```python
from build123d import *

# Parameters (mm, degrees)
CROQUIS1_W                     = 0.64
CROQUIS1_H                     = 0.64
SALIENTE_EXTRUIR1_DEPTH        = 2.54
SALIENTE_EXTRUIR2_DEPTH        = 8.54
SALIENTE_EXTRUIR2_DEPTH_BACK   = 3
CROQUIS3_W                     = 0.64
CROQUIS3_H                     = 0.64
SALIENTE_EXTRUIR2_2_DEPTH      = 8.54
SALIENTE_EXTRUIR2_2_DEPTH_BACK = 3
CHAFL_N1_SIZE                  = 0.2
CHAFL_N2_SIZE                  = 0.2
CROQUIS1_4_W                   = 11
CROQUIS1_4_H                   = 3
BOSS_EXTRUDE6_DEPTH            = 2.54
SKETCH6_W                      = 11
SKETCH6_H                      = 3
SKETCH6_R                      = 1
BOSS_EXTRUDE11_DEPTH           = 0.8
SKETCH7_W                      = 13
SKETCH7_H                      = 5
SKETCH7_W_2                    = 11
SKETCH7_H_2                    = 3
BOSS_EXTRUDE12_DEPTH           = 15
SKETCH8_W                      = 13
SKETCH8_H                      = 5
SKETCH8_R                      = 2
BOSS_EXTRUDE13_DEPTH           = 1
BOSS_EXTRUDE15_DEPTH           = 2
BOSS_EXTRUDE15_DEPTH_BACK      = 1.5
SKETCH9_R                      = 3
SKETCH9_R_2                    = 2
SKETCH10_W                     = 0.5
SKETCH10_H                     = 1.275200555
CUT_EXTRUDE2_DEPTH             = 3
BOSS_EXTRUDE20_DEPTH           = 3
CUT_EXTRUDE3_DEPTH             = 3
CUT_EXTRUDE5_DEPTH             = 18.878324866
CUT_EXTRUDE5_DEPTH_BACK        = 18.878324866


with BuildPart() as part:
    # Croquis1 → Saliente-Extruir1 (new body)
    # profile 1 of 2: a face of its own
    with BuildSketch(Plane(origin=(0, 0, 0), x_dir=(0, 0, -1), z_dir=(1, 0, 0))):
        Polygon((1.27, 0.595482683), (1.27, -0.595482683), (0.595482683, -1.27), (-0.595482683, -1.27), (-1.27, -0.595482683), (-1.27, 0.595482683), (-0.595482683, 1.27), (0.595482683, 1.27), align=None)
        Rectangle(CROQUIS1_W, CROQUIS1_H, mode=Mode.SUBTRACT)
    # profile 2 of 2: a face of its own
    with BuildSketch(Plane(origin=(0, 0, 0), x_dir=(0, 0, -1), z_dir=(1, 0, 0))):
        Polygon((3.135482683, 1.27), (3.81, 0.595482683), (3.81, -0.595482683), (3.135482683, -1.27), (1.944517317, -1.27), (1.27, -0.595482683), (1.27, 0.595482683), (1.944517317, 1.27), align=None)
        with Locations((2.54, 0)):
            Rectangle(CROQUIS1_W, CROQUIS1_H, mode=Mode.SUBTRACT)
    extrude(amount=SALIENTE_EXTRUIR1_DEPTH)

    # Mirror5: part across plane


with BuildPart() as body_2:
    # Croquis3 → Saliente-Extruir2 (new, two sides: drawn at the far end of the back side and taken through both)
    with BuildSketch(Plane(origin=(0, 0, 0), x_dir=(0, 0, -1), z_dir=(1, 0, 0)).offset(-SALIENTE_EXTRUIR2_DEPTH_BACK)):
        Rectangle(CROQUIS3_W, CROQUIS3_H)
    extrude(amount=SALIENTE_EXTRUIR2_DEPTH + SALIENTE_EXTRUIR2_DEPTH_BACK)

    # Chaflán1
    chafl_n1_edges = [body_2.edges().sort_by_distance(p)[0] for p in [
        (-3, 0, -0.32),
        (8.54, 0, 0.32),
        (8.54, -0.32, 0),
        (-3, 0.32, 0),
        (8.54, 0, -0.32),
        (8.54, 0.32, 0),
        (-3, 0, 0.32),
        (-3, -0.32, 0),
    ]]
    chamfer(chafl_n1_edges, length=CHAFL_N1_SIZE)


with BuildPart() as body_3:
    # Croquis3 → Saliente-Extruir2 2 (new, two sides: drawn at the far end of the back side and taken through both)
    with BuildSketch(Plane(origin=(0, 0, 0), x_dir=(0, 0, -1), z_dir=(1, 0, 0)).offset(-SALIENTE_EXTRUIR2_2_DEPTH_BACK)):
        with Locations((2.54, 0)):
            Rectangle(CROQUIS3_W, CROQUIS3_H)
    extrude(amount=SALIENTE_EXTRUIR2_2_DEPTH + SALIENTE_EXTRUIR2_2_DEPTH_BACK)

    # Chaflán2
    chafl_n2_edges = [body_3.edges().sort_by_distance(p)[0] for p in [
        (-3, 0, -2.86),
        (8.54, 0, -2.22),
        (8.54, -0.32, -2.54),
        (-3, 0.32, -2.54),
        (8.54, 0, -2.86),
        (8.54, 0.32, -2.54),
        (-3, 0, -2.22),
        (-3, -0.32, -2.54),
    ]]
    chamfer(chafl_n2_edges, length=CHAFL_N2_SIZE)


with BuildPart() as body_4:
    # Mirror3: mirrored copy
    add(body_2.part.mirror(Plane(origin=(2.54, 0, 1.27), x_dir=(1, 0, 0), z_dir=(0, 0, -1))))


with BuildPart() as body_5:
    # Mirror3 2: mirrored copy
    add(body_3.part.mirror(Plane(origin=(2.54, 0, 1.27), x_dir=(1, 0, 0), z_dir=(0, 0, -1))))


with BuildPart() as part_1:
    add(part.part)
    add(part.part.mirror(Plane(origin=(2.54, 0, 1.27), x_dir=(1, 0, 0), z_dir=(0, 0, -1))))


with BuildPart() as body_6:
    # Croquis1<4> → Boss-Extrude6 (new body)
    with BuildSketch(Plane(origin=(0, 0, 0), x_dir=(0, 0, -1), z_dir=(1, 0, 0))):
        with Locations((-1.27, 0)):
            Rectangle(CROQUIS1_4_W, CROQUIS1_4_H)
        Polygon((1.944517317, 1.27), (3.135482683, 1.27), (3.81, 0.595482683), (3.81, -0.595482683), (3.135482683, -1.27), (1.944517317, -1.27), (1.27, -0.595482683), (0.595482683, -1.27), (-0.595482683, -1.27), (-1.27, -0.595482683), (-1.27, 0.595482683), (-0.595482683, 1.27), (0.595482683, 1.27), (1.27, 0.595482683), align=None, mode=Mode.SUBTRACT)
    extrude(amount=BOSS_EXTRUDE6_DEPTH)

    # Combine5: cut body 2, body 3, body 4, body 5, part
    add(body_2.part, mode=Mode.SUBTRACT)
    add(body_3.part, mode=Mode.SUBTRACT)
    add(body_4.part, mode=Mode.SUBTRACT)
    add(body_5.part, mode=Mode.SUBTRACT)
    add(part_1.part, mode=Mode.SUBTRACT)

    # Sketch6 → Boss-Extrude11 (add)
    with BuildSketch(Plane.ZY):
        with Locations((1.27, 0)):
            Rectangle(SKETCH6_W, SKETCH6_H)
        with Locations((-2.54, 0)):
            Circle(SKETCH6_R, mode=Mode.SUBTRACT)
        with Locations((0, 0.013602928)):
            Circle(SKETCH6_R, mode=Mode.SUBTRACT)
        with Locations(Location((2.54, 0, 0), (0, 0, 180))):
            Circle(SKETCH6_R, mode=Mode.SUBTRACT)
        with Locations(Location((5.08, 0, 0), (0, 0, 180))):
            Circle(SKETCH6_R, mode=Mode.SUBTRACT)
    extrude(amount=BOSS_EXTRUDE11_DEPTH)

    # Sketch7 → Boss-Extrude12 (add)
    with BuildSketch(Plane(origin=(2.54, 0, 0), x_dir=(0, 0, -1), z_dir=(1, 0, 0))):
        with Locations((-1.27, 0)):
            Rectangle(SKETCH7_W, SKETCH7_H)
        with Locations((-1.27, 0)):
            Rectangle(SKETCH7_W_2, SKETCH7_H_2, mode=Mode.SUBTRACT)
    extrude(amount=-BOSS_EXTRUDE12_DEPTH)

    # Sketch8 → Boss-Extrude13 (add)
    with BuildSketch(Plane.ZY.offset(12.46)):
        with Locations((1.27, 0)):
            Rectangle(SKETCH8_W, SKETCH8_H)
        with Locations(Location((1.27, 0, 0), (0, 0, 131.409622109))):
            Circle(SKETCH8_R, mode=Mode.SUBTRACT)
    extrude(amount=BOSS_EXTRUDE13_DEPTH)

    # Sketch9 → Boss-Extrude15 (add, two sides: drawn at the far end of the back side and taken through both)
    with BuildSketch(Plane.ZY.offset(13.46).offset(-BOSS_EXTRUDE15_DEPTH_BACK)):
        with Locations(Location((1.27, 0, 0), (0, 0, 123.557309762))):
            Circle(SKETCH9_R)
        with Locations(Location((1.27, 0, 0), (0, 0, 131.409622109))):
            Circle(SKETCH9_R_2, mode=Mode.SUBTRACT)
    extrude(amount=BOSS_EXTRUDE15_DEPTH + BOSS_EXTRUDE15_DEPTH_BACK)

    # Sketch10 → Cut-Extrude2 (cut)
    with BuildSketch(Plane(origin=(0, -1.5, 0), x_dir=(1, 0, 0), z_dir=(0, 1, 0))):
        Polygon((-12.46, -3.868076211), (-12.46, -4.27), (-11.96, -4.27), (-10.789863612, -4.27), (-10.789863612, 1.73), (-12.46, 1.73), (-12.46, 1.328076211), (-11.96, 1.328076211), (-11.96, 0.052875656), (-12.46, 0.052875656), (-12.46, -2.592875656), (-11.96, -2.592875656), (-11.96, -3.868076211), align=None)
        with Locations((-12.21, -3.230475934)):
            Rectangle(SKETCH10_W, SKETCH10_H)
        with Locations((-12.21, 0.690475934)):
            Rectangle(SKETCH10_W, SKETCH10_H)
    extrude(amount=CUT_EXTRUDE2_DEPTH, mode=Mode.SUBTRACT)

    # Sketch15 → Boss-Extrude20 (add)
    with BuildSketch(Plane(origin=(-12.46, 0, 0), x_dir=(0, 0, -1), z_dir=(1, 0, 0))):
        with BuildLine():
            Line((4.23, -1.5), (4.23, 1.5))
            Line((4.23, 1.5), (0.052875656, 1.5))
            ThreePointArc((0.052875656, 1.5), (0.73, 0), (0.052875656, -1.5))
            Line((0.052875656, -1.5), (4.23, -1.5))
        make_face()
        with BuildLine():
            Line((-2.592875656, -1.5), (-6.77, -1.5))
            Line((-6.77, -1.5), (-6.77, 1.5))
            Line((-6.77, 1.5), (-2.592875656, 1.5))
            ThreePointArc((-2.592875656, 1.5), (-3.27, 0), (-2.592875656, -1.5))
        make_face()
    extrude(amount=BOSS_EXTRUDE20_DEPTH)

    # Sketch16 → Cut-Extrude3 (cut)
    with BuildSketch(Plane(origin=(0, 1.5, 0), x_dir=(1, 0, 0), z_dir=(0, 1, 0))):
        Polygon((-9.46, -2.592875656), (-12.46, -2.592875656), (-9.46, -6.77), align=None)
        Polygon((-12.46, 0.052875656), (-9.46, 4.23), (-9.46, 0.052875656), align=None)
    extrude(amount=-CUT_EXTRUDE3_DEPTH, mode=Mode.SUBTRACT)

    # Sketch19 → Cut-Extrude5 (cut, two sides: drawn at the far end of the back side and taken through both)
    with BuildSketch(Plane(origin=(0, 1.5, 0), x_dir=(1, 0, 0), z_dir=(0, 1, 0)).offset(-CUT_EXTRUDE5_DEPTH_BACK)):
        Polygon((-13.46, 5.23), (-9.957705311, 5.23), (-10.167106781, 4.937106781), (-12.46, 1.73), (-13.46, 1.73), align=None)
        Polygon((-13.46, -4.27), (-12.46, -4.27), (-10.167106781, -7.477106781), (-9.957705311, -7.77), (-13.46, -7.77), align=None)
    extrude(amount=CUT_EXTRUDE5_DEPTH + CUT_EXTRUDE5_DEPTH_BACK, mode=Mode.SUBTRACT)


solid = body_6.part
```
Part model, mm, in its own coordinate system. A direction names the side the tool comes from. Round coordinates to 2 decimals unless told otherwise and drop trailing zeros. Write each loop counter-clockwise with the first axis right and the second up, starting at its lowest first coordinate (ties: lowest second). Pieces come first, ordered by that corner, then holes.
Item 1: Cut at C-C, the plane z = -2.54. Give the cut face in (x, y).
Results:
outline: (-11.88, -2.5) - (2.54, -2.5) - (2.54, -1.27) - (0, -1.27) - (0, -1) - (-0.8, -1) - (-0.8, -1.5) - (-10.67, -1.5) - (-10.67, 1.5) - (-0.8, 1.5) - (-0.8, 1) - (0, 1) - (0, 1.27) - (2.54, 1.27) - (2.54, 2.5) - (-11.88, 2.5) - close
Item 2: Probe L1, parallel to Y at x = -9.75, z = 5.75; L2, parallel to Y at x = -14, z = 1.27; L3, parallel to Z at x = -5.5, y = 0.45. List the from-to ranges inside material, lowest first.
Results:
L1: y = -2.5 to -1.5, 1.5 to 2.5
L2: y = -3 to -2, 2 to 3
L3: z = -5.23 to -4.23, 6.77 to 7.77
Item 3: Which spindle directions (+Z, -Z, +X, -X, +Y, -Y) get a long thin tool onto all of the face, cutting with end or side? Do faces 1 (the flat face through (-13.46, -2, 4)), 2 (the flat face through (1, 1.27, 0)), 3 (the flat face through (-10.981, 0.021, -2.112)). Say none if no direction does.
Results:
face 1: +Z, -X, -Y
face 2: +X
face 3: none
Item 4: Cut at D-D, the plane y = 0.3. Count the separate pieces of the cut face and the enclosed holes in it, plus the area to 3 significant figures.
Results:
separate pieces: 5
enclosed holes: 0
area: 44.4 mm2
Item 5: Drop flat-ended pins along their axis: pin 1 Ø1.5 at (x, z) = (-10.5, 4.5) entering from +Y; pin 2 Ø2.5 at (x, z) = (-11.5, -2.5) entering from -Y; pin 3 Ø1.3 at (y, z) = (0, -0.5) entering from +X. Give the stop position or say it passes through.
Results:
pin 1: stops at y = 2.5
pin 2: stops at y = -2.5
pin 3: stops at x = 0
Item 6: Cut at B-B, the plane y = -2.25. Give the cut face in (x, z).
Results:
outline: (-15.46, -0.71) - (-13.46, -0.71) - (-13.46, -1.73) - (-12.46, -1.73) - (-9.96, -5.23) - (2.54, -5.23) - (2.54, 7.77) - (-9.96, 7.77) - (-12.46, 4.27) - (-13.46, 4.27) - (-13.46, 3.25) - (-15.46, 3.25) - close
Item 7: Two-plate mould, pull along Z, no slides. Class faces 4 (the flat face through (-13, 0, 4.27)), 5 (the flat face through (1, 1.27, 5)), 6 (the flat face through (-13.46, -1.9, -1.4)): +Z half, -Z half, draft (parallel to the pull), parting line (faces both ways), or undercut.
Results:
face 4: +Z half
face 5: undercut
face 6: draft
